```python
from build123d import *

# Parameters (mm, degrees)
SKETCH1_W           = 10
SKETCH1_H           = 10
BOSS_EXTRUDE1_DEPTH = 20
BOSS_EXTRUDE2_DEPTH = 10


with BuildPart() as part:
    # Sketch1 → Boss-Extrude1 (new body)
    with BuildSketch(Plane.XY):
        Rectangle(SKETCH1_W, SKETCH1_H)
    extrude(amount=BOSS_EXTRUDE1_DEPTH)

    # Sketch2 → Boss-Extrude2 (add)
    with BuildSketch(Plane.XY.offset(20)):
        with BuildLine():
            Line((0.956391162, 1.155558716), (1.0421378, -1.078864591))
            ThreePointArc((1.0421378, -1.078864591), (-1.498896721, -0.057520593), (0.956391162, 1.155558716))
        make_face()
    extrude(amount=BOSS_EXTRUDE2_DEPTH)


solid = part.part
```
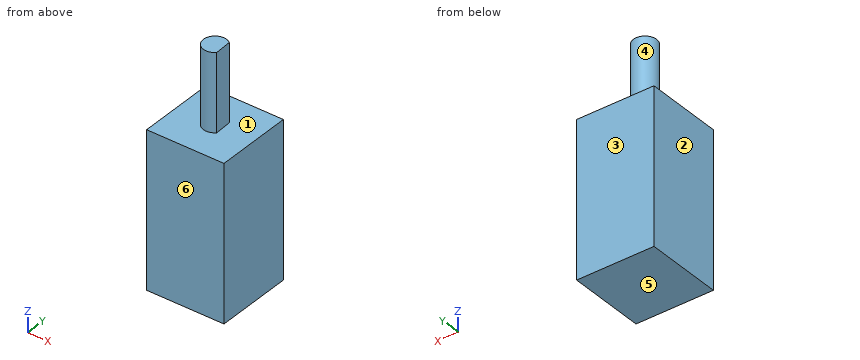
Design review of the part built by this model. Coordinates are the model's own, in mm. Face numbers are marked on the shaded views. A direction names the side the tool comes from. Coordinates: 2 decimals unless noted, no trailing zeros. Order: outer loops, then holes, each group sorted by start corner. A loop starts at its lowest first (then second) coordinate and runs counter-clockwise, first axis right, second up. Notation, with made-up numbers: (48, 20.5) -> (93, 20.5) arc R13 ccw to (93, 36.5) -> close; hole circle Ø1 at (-6.75, 13). An arc over 180 degrees is marked (long way). One line per item, written item: value. Start each with the question number.
Q1. Insertion check: pin 1 Ø2 at (x, y) = (-1.5, 3.5) entering from +Z; pin 2 Ø3 at (x, z) = (-1.5, 26.5) entering from -Y. Each pin has a flat end and moves straight along its axis. Give the tip position at first contact, or say it passes through.
Q2. Take a section at D-D, the plane y = 0. State the section outline as (x, z) points.
Q3. Take a section at A-A, the plane x = 0. State the section outline as (y, z) points, then the cut area to 3 significant figures.
Q4. Take a section at C-C, the plane z = 21. State the section outline as (x, y) points, then the cut area to 3 significant figures.
Q5. Take a section at B-B, the plane y = 2.75. State the section outline as (x, z) points.
Q6. Mouldability with a two-part tool opening along Y and no side actions: class the marked faces 3, 4, 5 and 6 as pulls with the +Y half, pulls with the -Y half, needs draft (parallel to the pull), parting line crosses it, or undercut.
Q7. For probe 1 along Z at (x, y) = (-2.5, -4); probe 2 along X at (y, z) = (1.25, 23.25), list the stretches that pass through material, from the lowest coordinate up.
Q8. Tool access review of the marked faces 1 and 2: name each direction out of +Z, -Z, +X, -X, +Y, -Y from which nothing blocks a thin tool from reaching the whole face with its end or side.
Values follow:
1. pin 1: stops at z = 20
1. pin 2: stops at y = -1.5
2. outline: (-5, 0) -> (5, 0) -> (5, 20) -> (1, 20) -> (1, 30) -> (-1.5, 30) -> (-1.5, 20) -> (-5, 20) -> close
3. outline: (-5, 0) -> (5, 0) -> (5, 20) -> (1.5, 20) -> (1.5, 30) -> (-1.5, 30) -> (-1.5, 20) -> (-5, 20) -> close
3. area: 230 mm2
4. outline: (0.96, 1.16) arc R1.5 ccw (long way) to (1.04, -1.08) -> close
4. area: 6.29 mm2
5. outline: (-5, 0) -> (5, 0) -> (5, 20) -> (-5, 20) -> close
6. face 3: pulls with the +Y half
6. face 4: parting line crosses it
6. face 5: needs draft
6. face 6: pulls with the -Y half
7. probe 1: z = 0 to 20
7. probe 2: x = -0.83 to 0.83
8. face 1: +Z
8. face 2: +Z, -Z, -X, +Y, -Y
